For this review, take the finished solid that the model builds, in its own axes (mm). A direction names the side the tool comes from. Round coordinates to 2 decimals unless told otherwise and drop trailing zeros. Order: outer loops, then holes, each group sorted by start corner. A loop starts at its lowest first (then second) coordinate and runs counter-clockwise, first axis right, second up.
from build123d import *
from OCP.BRepFilletAPI import BRepFilletAPI_MakeChamfer

# Parameters (mm, degrees)
SKETCH1_R           = 12
SKETCH1_R_2         = 10
BOSS_EXTRUDE1_DEPTH = 298
SKETCH2_R           = 14
SKETCH2_R_2         = 10
BOSS_EXTRUDE2_DEPTH = 15
SKETCH4_W           = 12
SKETCH4_H           = 7.5
CUT_EXTRUDE1_DEPTH  = 1
SKETCH5_R           = 2.5
CUT_EXTRUDE2_DEPTH  = 5
SKETCH6_R           = 11
BOSS_EXTRUDE3_DEPTH = 0.75
SKETCH7_R           = 10
BOSS_EXTRUDE4_DEPTH = 12
SKETCH9_R           = 14
SKETCH9_R_2         = 10
BOSS_EXTRUDE6_DEPTH = 15
SKETCH10_R          = 11
BOSS_EXTRUDE7_DEPTH = 0.75
SKETCH11_R          = 10
BOSS_EXTRUDE8_DEPTH = 20
CUT_EXTRUDE4_DEPTH  = 20
SKETCH13_R          = 3
CUT_EXTRUDE5_DEPTH  = 327.758798668
SKETCH14_R          = 4.5
CUT_EXTRUDE6_DEPTH  = 70
CHAMFER1_SIZE       = 1
CHAMFER1_SIZE2      = 0.176326981


with BuildPart() as part:
    # Sketch1 → Boss-Extrude1 (new body)
    with BuildSketch(Plane(origin=(0, 0, 0), x_dir=(1, 0, 0), z_dir=(0, 1, 0))):
        with Locations(Location((0, 0, 0), (0, 0, 270))):
            Circle(SKETCH1_R)
        with Locations(Location((0, 0, 0), (0, 0, 270))):
            Circle(SKETCH1_R_2, mode=Mode.SUBTRACT)
    extrude(amount=BOSS_EXTRUDE1_DEPTH)

    # Sketch2 → Boss-Extrude2 (add)
    with BuildSketch(Plane(origin=(0, 298, 0), x_dir=(1, 0, 0), z_dir=(0, 1, 0))):
        with Locations(Location((0, 0, 0), (0, 0, 270))):
            Circle(SKETCH2_R)
        with Locations(Location((0, 0, 0), (0, 0, 270))):
            Circle(SKETCH2_R_2, mode=Mode.SUBTRACT)
    extrude(amount=BOSS_EXTRUDE2_DEPTH)

    # Sketch4 → Cut-Extrude1 (cut)
    with BuildSketch(Plane(origin=(11.289405747, 313, 8.279451545), x_dir=(0.5913893960477971, 0, -0.8063861247828004), z_dir=(0.8063861247828003, 0, 0.591389396047797))):
        with Locations((0, -3.75)):
            Rectangle(SKETCH4_W, SKETCH4_H)
    cut_extrude1 = extrude(amount=-CUT_EXTRUDE1_DEPTH, mode=Mode.SUBTRACT)

    # Mirror1: Cut-Extrude1 across plane
    add(cut_extrude1.mirror(Plane(origin=(0, 313, 0), x_dir=(-0.5913893960477972, 0, 0.8063861247828003), z_dir=(0.8063861247828004, 0, 0.5913893960477971))), mode=Mode.SUBTRACT)

    # Sketch5 → Cut-Extrude2 (cut)
    with BuildSketch(Plane(origin=(-9.547499861, 313, 10.239396779), x_dir=(0.7313854842378409, 0, 0.6819642757844279), z_dir=(-0.6819642757844279, 0, 0.7313854842378409))):
        with Locations((0, -8)):
            Circle(SKETCH5_R)
    extrude(amount=-CUT_EXTRUDE2_DEPTH, mode=Mode.SUBTRACT)

    # Sketch6 → Boss-Extrude3 (add)
    with BuildSketch(Plane(origin=(0, 313, 0), x_dir=(1, 0, 0), z_dir=(0, 1, 0))):
        with Locations(Location((0, 0, 0), (0, 0, 270))):
            Circle(SKETCH6_R)
    extrude(amount=BOSS_EXTRUDE3_DEPTH)

    # Sketch7 → Boss-Extrude4 (add)
    with BuildSketch(Plane(origin=(0, 313.75, 0), x_dir=(1, 0, 0), z_dir=(0, 1, 0))):
        with Locations(Location((0, 0, 0), (0, 0, 270))):
            Circle(SKETCH7_R)
    extrude(amount=BOSS_EXTRUDE4_DEPTH)

    # Sketch9 → Boss-Extrude6 (add)
    with BuildSketch(Plane.XZ):
        with Locations(Location((0, 0, 0), (0, 0, 238.042455368))):
            Circle(SKETCH9_R)
        with Locations(Location((0, 0, 0), (0, 0, 270))):
            Circle(SKETCH9_R_2, mode=Mode.SUBTRACT)
    extrude(amount=BOSS_EXTRUDE6_DEPTH)

    # Sketch10 → Boss-Extrude7 (add)
    with BuildSketch(Plane.XZ.offset(15)):
        with Locations(Location((0, 0, 0), (0, 0, 90))):
            Circle(SKETCH10_R)
    extrude(amount=BOSS_EXTRUDE7_DEPTH)

    # Sketch11 → Boss-Extrude8 (add)
    with BuildSketch(Plane.XZ.offset(15.75)):
        with Locations(Location((0, 0, 0), (0, 0, 270))):
            Circle(SKETCH11_R)
    extrude(amount=BOSS_EXTRUDE8_DEPTH)

    # Sketch12 → Cut-Extrude4 (cut)
    with BuildSketch(Plane.XZ.offset(35.75)):
        with BuildLine():
            Line((-7.5, -6.614378278), (-7.5, 6.614378278))
            ThreePointArc((-7.5, 6.614378278), (-10, 0), (-7.5, -6.614378278))
        make_face()
        with BuildLine():
            ThreePointArc((10, 0), (9.354143467, 3.535533906), (7.5, 6.614378278))
            Line((7.5, 6.614378278), (7.5, -6.614378278))
            ThreePointArc((7.5, -6.614378278), (9.354143467, -3.535533906), (10, 0))
        make_face()
    extrude(amount=-CUT_EXTRUDE4_DEPTH, mode=Mode.SUBTRACT)

    # Sketch13 → Cut-Extrude5 (cut, through all)
    with BuildSketch(Plane(origin=(7.5, 0, 0), x_dir=(0, 0, -1), z_dir=(1, 0, 0))):
        with Locations((0, -26.75)):
            Circle(SKETCH13_R)
    extrude(amount=-CUT_EXTRUDE5_DEPTH, mode=Mode.SUBTRACT)

    # Sketch14 → Cut-Extrude6 (cut)
    with BuildSketch(Plane(origin=(0, 325.75, 0), x_dir=(1, 0, 0), z_dir=(0, 1, 0))):
        with Locations(Location((0, 0, 0), (0, 0, 270))):
            Circle(SKETCH14_R)
    extrude(amount=-CUT_EXTRUDE6_DEPTH, mode=Mode.SUBTRACT)

    # Chamfer1: one chamfer whose edges measure the first distance from different faces: ONE call of the kernel's chamfer builder (chamfer() names one face for all edges)
    chamfer1_edges_1 = [part.edges().sort_by_distance(p)[0] for p in [
        (0, 313, -4.5),
    ]]
    chamfer1_side_1 = [part.faces().sort_by_distance(p)[0] for p in [
        (0, 319.375, -4.5),
    ]]
    chamfer1_edges_2 = [part.edges().sort_by_distance(p)[0] for p in [
        (0, 325.75, -4.5),
    ]]
    chamfer1_side_2 = [part.faces().sort_by_distance(p)[0] for p in [
        (0, 325.75, -9.717157288),
    ]]
    chamfer1_edges_3 = [part.edges().sort_by_distance(p)[0] for p in [
        (0, 325.75, -10),
    ]]
    chamfer1_side_3 = [part.faces().sort_by_distance(p)[0] for p in [
        (0, 319.75, -10),
    ]]
    chamfer1 = BRepFilletAPI_MakeChamfer(part.part.solid().wrapped)
    for e in chamfer1_edges_1:
        chamfer1.Add(CHAMFER1_SIZE, CHAMFER1_SIZE2, e.wrapped, chamfer1_side_1[0].wrapped)  # the first distance lies on this face
    for e in chamfer1_edges_2:
        chamfer1.Add(CHAMFER1_SIZE, CHAMFER1_SIZE2, e.wrapped, chamfer1_side_2[0].wrapped)  # the first distance lies on this face
    for e in chamfer1_edges_3:
        chamfer1.Add(CHAMFER1_SIZE, CHAMFER1_SIZE2, e.wrapped, chamfer1_side_3[0].wrapped)  # the first distance lies on this face
    add(Compound.cast(chamfer1.Shape()), mode=Mode.REPLACE)


solid = part.part
(1) Clearance check with flat-ended pins moving along their axes: P1, Ø5, axis at y = 69, z = 3, coming from the +X side; P2, Ø12, axis at x = 9, y = 193.5, coming from the -Z side; P3, Ø8, axis at x = -2, y = 225.5, coming from the +Z side. State where each tip first meets the part, or that it passes through.
(2) Add section A-A on y = -26.75. Give the boundary of the cut face in (x, z).
(3) Tool access review of faces 1 (the face through (0, -26, 10)), 2 (the face through (11, 305.5, 8)), 3 (the face through (-10, 313.75, 2)), 4 (the face through (10.4, 298, -6.3)): name each direction out of +Z, -Z, +X, -X, +Y, -Y from which nothing blocks a thin tool from reaching the whole face with its end or side.
(4) Wall thickness on L1, parallel to X at y = 178, z = 0; L2, parallel to X at y = 321.5, z = 0; L3, parallel to Y at x = -5.5, z = 5.75: over which ranges is each line inside the solid? List them lowest first.
(5) Add section B-B on y = 228. Give the boundary of the cut face in (x, z).
(6) Draft analysis for pull direction Y (two halves, no side actions). For faces 5 (the face through (0, -15, 0)), 6 (the face through (8, -15.75, 1)), 7 (the face through (0, -26, -10)), state which applies: pulls with the +Y half, pulls with the -Y half, needs draft (parallel to the pull), parting line crosses it, or undercut.
Here are the results:
1. P1: stops at x = 11.99
1. P2: stops at z = -11.62
1. P3: stops at z = 12
2. outline: (-7.5, -6.61) arc R10 ccw to (7.5, -6.61) - (7.5, -3) - (-7.5, -3) - close; (-7.5, 3) - (7.5, 3) - (7.5, 6.61) arc R10 ccw to (-7.5, 6.61) - close
3. face 1: +Z, -Y
3. face 2: +Z, +X, +Y
3. face 3: +Y
3. face 4: none
4. L1: x = -12 to -10, 10 to 12
4. L2: x = -10 to -4.5, 4.5 to 10
4. L3: y = -35.75 to -15, 313 to 325.75
5. outline: circle Ø24 at (0, 0); hole circle Ø20 at (0, 0)
6. face 5: undercut
6. face 6: pulls with the -Y half
6. face 7: needs draft
